Part model, mm, in its own coordinate system. A direction names the side the tool comes from. Give positions to 0.01 mm unless a question says otherwise; leave off trailing zeros. Write each loop counter-clockwise with the first axis right and the second up, starting at its lowest first coordinate (ties: lowest second). Pieces come first, ordered by that corner, then holes. Notation, with made-up numbers: (-9, -32.75) - (-3, -32.75) arc R21 cw to (-3, -23.75) - close; hole circle Ø7 at (35, 70). An arc over 180 degrees is marked (long way). Answer in a Markdown table with one row per item. Add a question column.
1. Drop a flat-ended pin along its axis: pin 1 Ø1 at (x, z) = (4.5, 0.5) entering from +Y. Give the stop position or say it passes through.
2. Probe line 1 along X through (y, z) = (0.4, -1.3); line 2 along Z through (x, y) = (0.5, 0.85); line 3 along Z through (x, y) = (10.5, -0.95). List the from-to ranges inside material, lowest first.
3. Band-saw the part on A-A on z = 0. Write the cut outline in (x, y).
4. Band-saw the part on C-C on x = 5. Write the cut outline in (y, z).
5. Which spindle directions (+Z, -Z, +X, -X, +Y, -Y) get a long thin tool onto all of the face, cutting with end or side? Do faces 1 (the cylindrical face through (0.6, -1.39, 0.31)), 2 (the cylindrical face through (5.85, 1, -0.63)). Say none if no direction does.
6. Band-saw the part on D-D on x = 1. Write the cut outline in (y, z), plus the area to 3 significant figures.
```python
from build123d import *

# Parameters (mm, degrees)
SKETCH1_R           = 1.4224
BOSS_EXTRUDE1_DEPTH = 1.2192
SKETCH2_R           = 1.1811
BOSS_EXTRUDE2_DEPTH = 9.652
CHAMFER1_SIZE       = 0.254
CHAMFER1_SIZE2      = 0.439940905


with BuildPart() as part:
    # Sketch1 → Boss-Extrude1 (new body)
    with BuildSketch(Plane(origin=(0, 0, 0), x_dir=(0, 0, -1), z_dir=(1, 0, 0))):
        Circle(SKETCH1_R)
    extrude(amount=BOSS_EXTRUDE1_DEPTH)

    # Sketch2 → Boss-Extrude2 (add)
    with BuildSketch(Plane(origin=(1.2192, 0, 0), x_dir=(0, 0, -1), z_dir=(1, 0, 0))):
        Circle(SKETCH2_R)
    extrude(amount=BOSS_EXTRUDE2_DEPTH)

    # Chamfer1
    chamfer1_edges = [part.edges().sort_by_distance(p)[0] for p in [
        (10.8712, 0, 1.1811),
    ]]
    chamfer1_side = [part.faces().sort_by_distance(p)[0] for p in [
        (6.0452, 0, 1.1811),
    ]]
    chamfer(chamfer1_edges, length=CHAMFER1_SIZE, length2=CHAMFER1_SIZE2, reference=chamfer1_side[0])


solid = part.part
```
Values:
| question | item | result |
|---|---|---|
| 1 | pin 1 | stops at y = 1.18 |
| 2 | line 1 | x = 0 to 1.22 |
| 2 | line 2 | z = -1.14 to 1.14 |
| 2 | line 3 | z = -0.7 to 0.7 |
| 3 | outline | (0, -1.42) - (1.22, -1.42) - (1.22, -1.18) - (10.62, -1.18) - (10.87, -0.74) - (10.87, 0.74) - (10.62, 1.18) - (1.22, 1.18) - (1.22, 1.42) - (0, 1.42) - close |
| 4 | outline | circle Ø2.36 at (0, 0) |
| 5 | face 1 | +X, -X |
| 5 | face 2 | +X |
| 6 | outline | circle Ø2.84 at (0, 0) |
| 6 | area | 6.36 mm² |
